Here's the drawing with two shaded views (mm, measured from the low corner). I have some questions. Round coordinates to 2 decimals unless told otherwise and drop trailing zeros. Order: outer loops, then holes, each group sorted by start corner. A loop starts at its lowest first (then second) coordinate and runs counter-clockwise, first axis right, second up. Notation, with made-up numbers: (7, -35.5) -> (60, -35.5) arc R34 ccw to (60, -2.5) -> close; hole circle Ø4 at (-10.5, 48). An arc over 180 degrees is marked (long way). Answer in a Markdown table with one row per item.
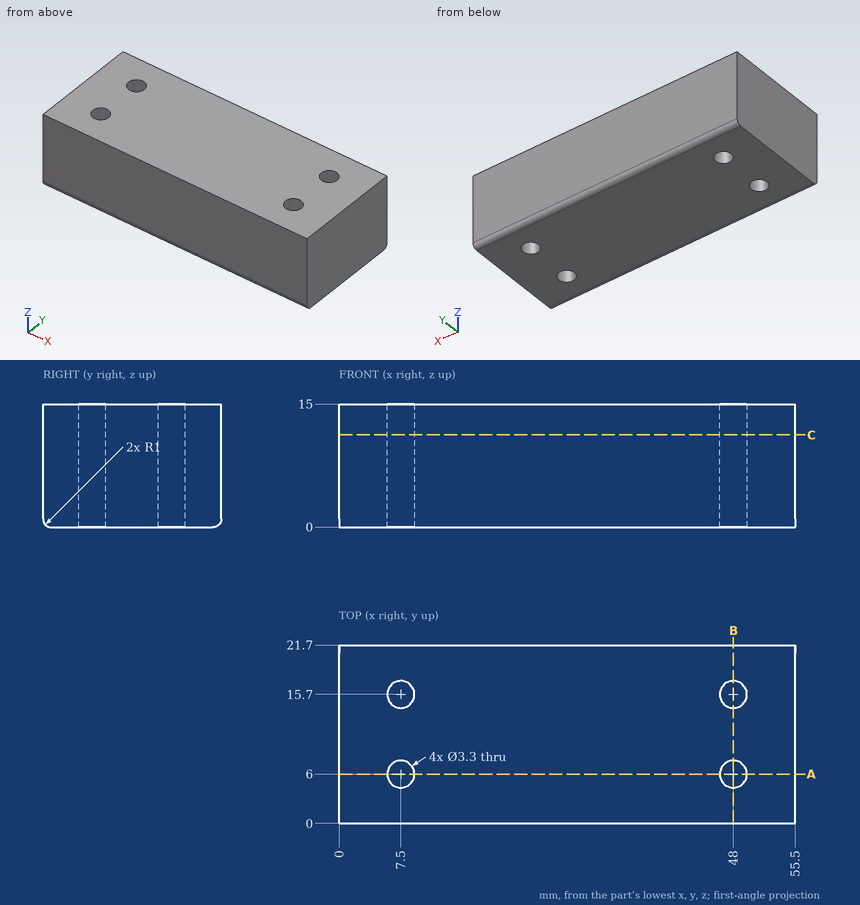
1. Suppose I cut it at B-B on x = 48. Write out the boundary of the cut face in (y, z).
Numbers:
| item | result |
|---|---|
| outline | (0, 1) arc R1 ccw to (1, 0) -> (4.35, 0) -> (4.35, 15) -> (0, 15) -> close; (7.65, 0) -> (14.05, 0) -> (14.05, 15) -> (7.65, 15) -> close; (17.35, 0) -> (20.7, 0) arc R1 ccw to (21.7, 1) -> (21.7, 15) -> (17.35, 15) -> close |
2. Suppose I cut it at A-A on y = 6. Write out the boundary of the cut face in (x, z), then the cut area to 4 significant figures.
Numbers:
| item | result |
|---|---|
| outline | (0, 0) -> (5.85, 0) -> (5.85, 15) -> (0, 15) -> close; (9.15, 0) -> (46.35, 0) -> (46.35, 15) -> (9.15, 15) -> close; (49.65, 0) -> (55.5, 0) -> (55.5, 15) -> (49.65, 15) -> close |
| area | 733.5 mm2 |
3. Suppose I cut it at C-C on z = 11.25. Write out the boundary of the cut face in (x, y), then the cut area to 3 significant figures.
Numbers:
| item | result |
|---|---|
| outline | (0, 0) -> (55.5, 0) -> (55.5, 21.7) -> (0, 21.7) -> close; hole circle Ø3.3 at (7.5, 6); hole circle Ø3.3 at (7.5, 15.7); hole circle Ø3.3 at (48, 6); hole circle Ø3.3 at (48, 15.7) |
| area | 1,170 mm2 |
4. Please list where these lines run through material, in increasing order: line 1 along Y through (x, z) = (48, 7.5); line 2 along X through (y, z) = (5.5, 13.75); line 3 along X through (y, z) = (14.5, 13.5).
Numbers:
| item | result |
|---|---|
| line 1 | y = 0 to 4.35, 7.65 to 14.05, 17.35 to 21.7 |
| line 2 | x = 0 to 5.93, 9.07 to 46.43, 49.57 to 55.5 |
| line 3 | x = 0 to 6.37, 8.63 to 46.87, 49.13 to 55.5 |
